For this review, take the finished solid that the model builds, in its own axes (mm). Face numbers are marked on the shaded views. A direction names the side the tool comes from. Coordinates: 2 decimals unless noted, no trailing zeros. Loops run counter-clockwise (first coordinate to the right, second up) from the corner with the lowest first, then second, coordinate; pieces in that order, holes last. Notation, with made-up numbers: M -23.5,-13.75 L 25.5,-13.75 A4 cw 25.5,-6.75 Z; hole C 9,45 d5. An arc over 180 degrees is marked long. Answer as a JSON object with one key per item and string values. Group by question number.
Item 1: Wall thickness on L1, parallel to Z at x = -5.25, y = -1.5; L2, parallel to X at y = -1.2, z = -2.5; L3, parallel to Z at x = 1.25, y = -0.95: over which ranges is each line inside the solid? List them lowest first. Write a range as from..to.
Item 2: Add section C-C (x = -4). State the section outline as (y, z) points, then the cut area to 3 significant figures.
Item 3: Add section B-B (x = 1). State the section outline as (y, z) points.
Item 4: Tool access review of the marked faces 4, 5, 6, 7 and 8: name each direction out of +Z, -Z, +X, -X, +Y, -Y from which nothing blocks a thin tool from reaching the whole face with its end or side.
Item 5: Mouldability with a two-part tool opening along Z and no side actions: class the marked faces 1, 2 and 3 as +Z half, -Z half, draft (parallel to the pull), parting line (faces both ways), or undercut.
Item 6: Add section A-A (y = -2.35). State the section outline as (x, z) points.
Item 7: Insertion check: pin 1 (1 mm diameter, centred on x = 2.5, y = -3.5, fed in from -Z); pin 2 (1.2 mm diameter, centred on y = -2, z = -3.5, fed in from -X); pin 3 (2.5 mm diameter, centred on y = -1.5, z = -2.5, fed in from +X). Each pin has a flat end and moves straight along its axis. Give the tip position at first contact, or say it passes through.
from build123d import *

# Parameters (mm, degrees)
F0_W     = 10
F0_H     = 5
F1_DEPTH = 16.999991
F2_W     = 5.999998
F2_H     = 2.499995
F3_DEPTH = 4.99872
F4_R     = 0.508


with BuildPart() as f1:
    # F0 (on Top) → F1 (new body)
    with BuildSketch(Plane.XY):
        with Locations((-1.278629, -2.023488)):
            Rectangle(F0_W, F0_H)
    extrude(amount=F1_DEPTH)

    # F2 (on face) → F3 (join)
    with BuildSketch(Plane(origin=(0, 0, 0), x_dir=(1, 0, 0), z_dir=(0, 0, -1))):
        with Locations((-1.278629, 2.023489)):
            Rectangle(F2_W, F2_H)
    extrude(amount=F3_DEPTH)

    # F4
    f4_edges = [f1.edges().sort_by_distance(p)[0] for p in [
        (-1.278629, -0.773491, 0),
        (1.72137, -2.023488, 0),
        (-4.278628, -2.023488, 0),
        (-1.278629, -3.273486, 0),
        (-4.278628, -2.023488, -4.99872),
        (1.72137, -2.023488, -4.99872),
        (3.721371, -2.023488, 0),
        (-1.278629, 0.476512, 0),
        (3.721371, 0.476512, 8.499996),
        (-6.278629, 0.476512, 8.499996),
        (-6.278629, -2.023488, 0),
        (-6.278629, -4.523488, 8.499996),
        (3.721371, -4.523488, 8.499996),
        (-1.278629, -4.523488, 0),
        (-1.278629, -4.523488, 16.999991),
        (-1.278629, 0.476512, 16.999991),
        (-6.278629, -2.023488, 16.999991),
        (3.721371, -2.023488, 16.999991),
    ]]
    fillet(f4_edges, radius=F4_R)


solid = f1.part
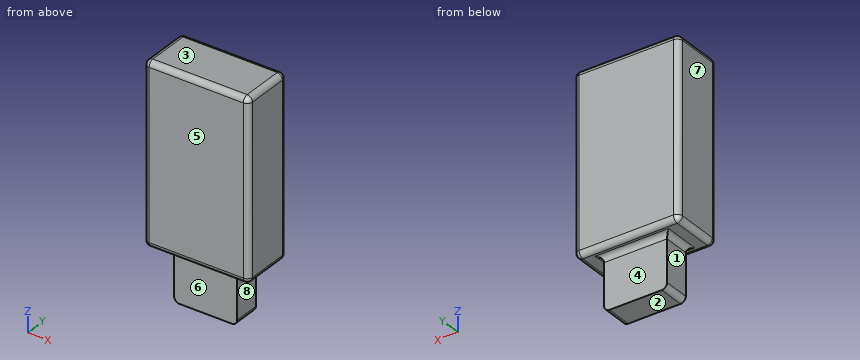
From the geometry:
{
 "1": {"L1": "z = 0..17", "L2": "x = -4.28..1.72", "L3": "z = -5..17"},
 "2": {"outline": "M -4.52,0.51 A0.51 ccw -4.02,0 L -3.78,0 A0.51 cw -3.27,-0.51 L -3.27,-4.94 L -0.77,-4.94 L -0.77,-0.51 A0.51 cw -0.27,0 L -0.03,0 A0.51 ccw 0.48,0.51 L 0.48,16.49 A0.51 ccw -0.03,17 L -4.02,17 A0.51 ccw -4.52,16.49 Z", "area": "97.2 mm²"},
 "3": {"outline": "M -4.52,0.51 A0.51 ccw -4.02,0 L -3.78,0 A0.51 cw -3.27,-0.51 L -3.27,-5 L -0.77,-5 L -0.77,-0.51 A0.51 cw -0.27,0 L -0.03,0 A0.51 ccw 0.48,0.51 L 0.48,16.49 A0.51 ccw -0.03,17 L -4.02,17 A0.51 ccw -4.52,16.49 Z"},
 "4": {"face 4": "-Z, +X, -X, +Y", "face 5": "+Z, -Z, +X, -X, -Y", "face 6": "-Z, +X, -X, -Y", "face 7": "+Z, -Z, -X, +Y, -Y", "face 8": "-Z, +X, +Y, -Y"},
 "5": {"face 1": "draft", "face 2": "-Z half", "face 3": "+Z half"},
 "6": {"outline": "M -6.28,0.51 A0.51 ccw -5.77,0 L -4.79,0 A0.51 cw -4.28,-0.51 L -4.28,-4.49 A0.51 ccw -3.77,-5 L 1.21,-5 A0.51 ccw 1.72,-4.49 L 1.72,-0.51 A0.51 cw 2.23,0 L 3.21,0 A0.51 ccw 3.72,0.51 L 3.72,16.49 A0.51 ccw 3.21,17 L -5.77,17 A0.51 ccw -6.28,16.49 Z"},
 "7": {"pin 1": "stops at z = -0.05", "pin 2": "stops at x = -4.28", "pin 3": "stops at x = 1.72"}
}
